Read the model definition and answer for the solid it produces. Units are mm, in the model's axes. Face numbers are marked on the shaded views. A direction names the side the tool comes from. Give positions to 0.01 mm unless a question says otherwise; leave off trailing zeros. Order: outer loops, then holes, each group sorted by start corner. A loop starts at its lowest first (then second) coordinate and runs counter-clockwise, first axis right, second up. Notation, with made-up numbers: M 86.5,-7.75 L 131.5,-7.75 A24 cw 131.5,11.25 Z; hole C 24.5,2 d6. An arc over 180 degrees is marked long. One line per item, written item: value.
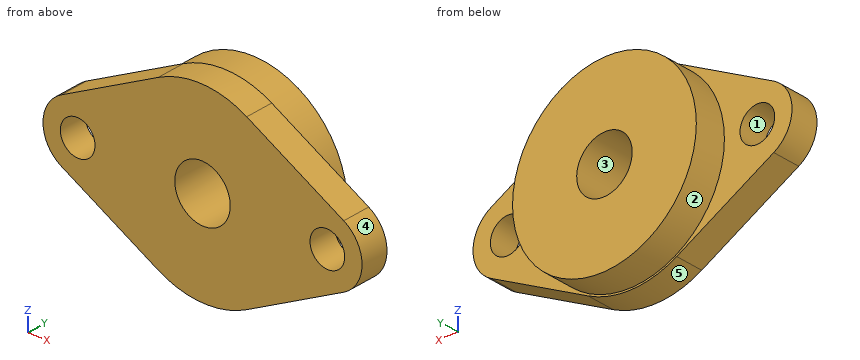
from build123d import *

# Parameters (mm, degrees)
SKETCH_1_R      = 4
SKETCH_1_R_2    = 2.5
EXTRUDE_1_DEPTH = 4
SKETCH_2_R      = 13.25
SKETCH_2_R_2    = 4
EXTRUDE_2_DEPTH = 4.5


with BuildPart() as part:
    # 草图1 → 凸台-拉伸1 (new body)
    with BuildSketch(Plane(origin=(0, 0, 0), x_dir=(1, 0, 0), z_dir=(0, 1, 0))):
        with BuildLine():
            Line((20.361111111, -4.407397681), (6.375, -11.899973739))
            ThreePointArc((6.375, -11.899973739), (0, -13.5), (-6.375, -11.899973739))
            Line((-6.375, -11.899973739), (-20.361111111, -4.407397681))
            ThreePointArc((-20.361111111, -4.407397681), (-23, 0), (-20.361111111, 4.407397681))
            Line((-20.361111111, 4.407397681), (-6.375, 11.899973739))
            ThreePointArc((-6.375, 11.899973739), (0, 13.5), (6.375, 11.899973739))
            Line((6.375, 11.899973739), (20.361111111, 4.407397681))
            ThreePointArc((20.361111111, 4.407397681), (23, 0), (20.361111111, -4.407397681))
        make_face()
        with Locations(Location((0, 0, 0), (0, 0, 270))):
            Circle(SKETCH_1_R, mode=Mode.SUBTRACT)
        with Locations(Location((18, 0, 0), (0, 0, 270))):
            Circle(SKETCH_1_R_2, mode=Mode.SUBTRACT)
        with Locations(Location((-18, 0, 0), (0, 0, 270))):
            Circle(SKETCH_1_R_2, mode=Mode.SUBTRACT)
    extrude(amount=EXTRUDE_1_DEPTH)

    # 草图2 → 凸台-拉伸2 (add)
    with BuildSketch(Plane(origin=(0, 4, 0), x_dir=(1, 0, 0), z_dir=(0, 1, 0))):
        with Locations(Location((0, 0, 0), (0, 0, 270))):
            Circle(SKETCH_2_R)
        with Locations(Location((0, 0, 0), (0, 0, 270))):
            Circle(SKETCH_2_R_2, mode=Mode.SUBTRACT)
    extrude(amount=EXTRUDE_2_DEPTH)


solid = part.part
1) Find section C-C, the plane y = 2.75. Write down the section's boundary in (x, z) (3 decimals), plus the area to 3 significant figures.
Reported:
outline: M -20.361,-4.407 L -6.375,-11.9 A13.5 ccw 6.375,-11.9 L 20.361,-4.407 A5 ccw 20.361,4.407 L 6.375,11.9 A13.5 ccw -6.375,11.9 L -20.361,4.407 A5 ccw Z; hole C -18,0 d5; hole C 0,0 d8; hole C 18,0 d5
area: 731 mm^2
2) Determine the mould class of the marked faces 3, 4 and 5 for opening direction Z: +Z half, -Z half, draft (parallel to the pull), parting line (faces both ways), or undercut.
Reported:
face 3: undercut
face 4: parting line
face 5: -Z half
3) Find section A-A, the plane x = 0. Write down the section's boundary in (y, z), plus the area to 3 significant figures.
Reported:
outline: M 0,-13.5 L 4,-13.5 L 4,-13.25 L 8.5,-13.25 L 8.5,-4 L 0,-4 Z; M 0,4 L 8.5,4 L 8.5,13.25 L 4,13.25 L 4,13.5 L 0,13.5 Z
area: 159 mm^2
4) Consider probe 1 along X at (y, z) = (7.5, -0.25); probe 2 along Z at (x, y) = (-16, 2.5); probe 3 along X at (y, z) = (6, 3). Determine where each line is inside the solid, lowest interval first.
Reported:
probe 1: x = -13.25 to -3.99, 3.99 to 13.25
probe 2: z = -6.74 to -1.5, 1.5 to 6.74
probe 3: x = -12.91 to -2.65, 2.65 to 12.91
5) Find section D-D, the plane z = 5. Write down the section's boundary in (x, y).
Reported:
outline: M -19.25,0 L 19.25,0 L 19.25,4 L 12.27,4 L 12.27,8.5 L -12.27,8.5 L -12.27,4 L -19.25,4 Z
6) Each of these flat-tipped pins is pushed along its axis until it touches: pin 1 Ø3 at (x, y) = (10, 6) entering from +Z; pin 2 Ø2 at (y, z) = (4, -5) entering from -X; pin 3 Ø3 at (x, y) = (-4.5, 1.5) entering from -Z. Where does it stop, or does it pass through?
Reported:
pin 1: stops at z = 10.16
pin 2: stops at x = -21
pin 3: stops at z = -13.16
7) Which of the six approach directions +Z, -Z, +X, -X, +Y, -Y give full straight-line access (tool end or side, diameter ignored) to the marked faces 1 and 2?
Reported:
face 1: +Y, -Y
face 2: +Y
8) Find section B-B, the plane z = 0. Write down the section's boundary in (x, y), plus the area to 3 significant figures.
Reported:
outline: M -23,0 L -20.5,0 L -20.5,4 L -23,4 Z; M -15.5,0 L -4,0 L -4,8.5 L -13.25,8.5 L -13.25,4 L -15.5,4 Z; M 4,0 L 15.5,0 L 15.5,4 L 13.25,4 L 13.25,8.5 L 4,8.5 Z; M 20.5,0 L 23,0 L 23,4 L 20.5,4 Z
area: 195 mm^2
